Autodesk Inventor part; units mm, degrees
ref_plane "YZ Plane" through (0, 0, 0) normal (1, 0, 0) x (0, 1, 0)
ref_plane "XZ Plane" through (0, 0, 0) normal (0, 1, 0) x (-1, 0, 0)
ref_plane "XY Plane" through (0, 0, 0) normal (0, 0, 1) x (1, 0, 0)
sketch "Sketch1" plane through (0, 0, 0) normal (0, 1, 0) x (-1, 0, 0)
  circle A0 centre (0, 0) radius 41.5
  circle A1 centre (0, 0) radius 36.5
  dimension "d0" = 83
  dimension "d1" = 73
extrude "Extrusion1" add sketch "Sketch1" along normal blind 2
sketch "Sketch4" plane through (0, 0, 0) normal (0, -1, 0) x (1, 0, 0)
  line L0 (-2.5, -20) -> (-2.5, -41.5)
  line L1 (-2.5, -41.5) -> (2.5, -41.5)
  line L2 (2.5, -41.5) -> (2.5, -20)
  line L3 (3.2204, 53.4593) -> (-2.5, -41.5) construction
  line L4 (-3.2204, 53.4593) -> (2.5, -41.5) construction
  line L5 (2.5, -20) -> (-2.5, -20)
  line L6 (41.5, 2.5) -> (20, 2.5)
  line L7 (20, -2.5) -> (41.5, -2.5)
  line L8 (20, 2.5) -> (20, -2.5)
  line L9 (41.5, -2.5) -> (41.5, 2.5)
  line L10 (-2.5, 41.5) -> (-2.5, 20)
  line L11 (2.5, 20) -> (2.5, 41.5)
  line L12 (-2.5, 20) -> (2.5, 20)
  line L13 (2.5, 41.5) -> (-2.5, 41.5)
  line L14 (-41.5, -2.5) -> (-20, -2.5)
  line L15 (-20, 2.5) -> (-41.5, 2.5)
  line L16 (-20, -2.5) -> (-20, 2.5)
  line L17 (-41.5, 2.5) -> (-41.5, -2.5)
  point P0 (0, 0)
  dimension "d21" = 5
  dimension "d26" = 360
  dimension "d51" = 20
  dimension "d52" = 41.5
extrude "Extrusion3" add sketch "Sketch4" along normal blind 3
sketch "Sketch5" plane through (0, -3, 0) normal (0, -1, 0) x (1, 0, 0)
  arc A0 (-41.4246, 2.5) -> (2.5, -41.4246) centre (0, 0) ccw
  line L0 (2.5, -41.4246) -> (-2.5, -41.4246)
  line L1 (-2.5, -41.4246) -> (-2.5, -36.9246)
  line L2 (-2.5, -36.9246) -> (2.5, -36.9246)
  line L3 (2.5, -36.9246) -> (2.5, -41.4246)
  line L4 (41.4246, 2.5) -> (41.4246, -2.5)
  line L5 (41.4246, -2.5) -> (36.9246, -2.5)
  line L6 (36.9246, -2.5) -> (36.9246, 2.5)
  line L7 (36.9246, 2.5) -> (41.4246, 2.5)
  line L8 (-2.5, 41.4246) -> (2.5, 41.4246)
  line L9 (2.5, 41.4246) -> (2.5, 36.9246)
  line L10 (2.5, 36.9246) -> (-2.5, 36.9246)
  line L11 (-2.5, 36.9246) -> (-2.5, 41.4246)
  line L12 (-41.4246, -2.5) -> (-41.4246, 2.5)
  line L13 (-41.4246, 2.5) -> (-36.9246, 2.5)
  line L14 (-36.9246, 2.5) -> (-36.9246, -2.5)
  line L15 (-36.9246, -2.5) -> (-41.4246, -2.5)
  point P0 (0, -41.5)
  dimension "d30" = 5
  dimension "d31" = 4.5
  dimension "d34" = 360
extrude "Extrusion4" add sketch "Sketch5" along normal blind 40 contours L13 L14 L15 L12 | L1 L2 L3 L0 | L4 L5 L6 L7 | L8 L9 L10 L11
sketch "Sketch7" plane through (0, 2, 0) normal (0, 1, 0) x (1, 0, 0)
  circle A0 centre (0, -39) radius 1.5
  circle A1 centre (0, -44.5) radius 1.5
  circle A2 centre (38.5381, -22.25) radius 1.5
  circle A3 centre (33.775, -19.5) radius 1.5
  circle A4 centre (38.5381, 22.25) radius 1.5
  circle A5 centre (33.775, 19.5) radius 1.5
  circle A6 centre (0, 44.5) radius 1.5
  circle A7 centre (0, 39) radius 1.5
  circle A8 centre (-38.5381, 22.25) radius 1.5
  circle A9 centre (-33.775, 19.5) radius 1.5
  circle A10 centre (-38.5381, -22.25) radius 1.5
  circle A11 centre (-33.775, -19.5) radius 1.5
  point P0 (0, 0)
  dimension "d41" = 3
  dimension "d42" = 39
  dimension "d43" = 3
  dimension "d44" = 44.5
  dimension "d47" = 360
extrude "Extrusion6" cut sketch "Sketch7" against normal blind 10 contours A2 | A3 | A4 | A5 | A8 | A9 | A10 | A11
sketch "Sketch8" plane through (0, -43, 0) normal (0, -1, 0) x (1, 0, 0)
  line L0 (-2.5, 36.4143) -> (-2.5, 41.4246)
  arc A0 (0, -41.5) -> (2.5, -41.4246) centre (0, 0) ccw
  line L1 (-2.5, 41.4246) -> (2.5, 41.4246)
  line L2 (2.5, 41.4246) -> (2.5, -41.4246)
  line L3 (2.5, -41.4246) -> (-2.5, -41.4246)
  line L4 (-2.5, -41.4246) -> (-2.5, 41.4246)
  line L5 (-36.4143, -2.5) -> (-41.4246, -2.5)
  line L6 (36.4143, 2.5) -> (41.4246, 2.5)
  line L7 (-41.4246, -2.5) -> (41.4246, -2.5)
  line L8 (41.4246, -2.5) -> (41.4246, 2.5)
  line L9 (41.4246, 2.5) -> (-41.4246, 2.5)
  line L10 (-41.4246, 2.5) -> (-41.4246, -2.5)
extrude "Extrusion7" add sketch "Sketch8" along normal blind 5
properties part number "Bottom- Control Surfaces"
Work out the finished part from the listing and answer in its coordinate system (mm). A direction names the side the tool comes from. Coordinates: 2 decimals unless noted, no trailing zeros. Loops run counter-clockwise (first coordinate to the right, second up) from the corner with the lowest first, then second, coordinate; pieces in that order, holes last. Notation, with made-up numbers: (82.25, -40) - (99.25, -40) arc R32 ccw to (99.25, -12) - close; hole circle Ø9 at (-12.75, 57.5). An arc over 180 degrees is marked (long way). Use a Markdown table: item, result.
Item 1: Consider probe 1 along Z at (x, y) = (0, 1); probe 2 along X at (y, z) = (1.35, -19.5) (1 decimal). Determine where each line is inside the solid, lowest interval first. Write a range as from..to.
Evaluation:
| item | result |
|---|---|
| probe 1 | z = -41.5..-36.5, 36.5..41.5 |
| probe 2 | x = -36.6..-35.3, -32.3..-30.9, 30.9..32.3, 35.3..36.6 |
Item 2: The mould has two halves that part along Z. Classify faces 1 (the cylindrical face through (-34.881, 1.014, -20.514)), 2 (the flat face through (41.425, -25, 0)), 3 (the flat face through (-38, -31, -2.5)): +Z half, -Z half, draft (parallel to the pull), parting line (faces both ways), or undercut.
Evaluation:
| item | result |
|---|---|
| face 1 | undercut |
| face 2 | draft |
| face 3 | -Z half |
Item 3: Given pin 1 Ø3 at (y, z) = (-4, -30) entering from -X; pin 2 Ø1.5 at (x, z) = (1, 26.5) entering from +Y; pin 3 Ø1 at (x, z) = (-30, -21) entering from -Y, each flat-ended and moving along its own axis, determine where each tip first touches the part or whether it passes through.
Evaluation:
| item | result |
|---|---|
| pin 1 | stops at x = -2.5 |
| pin 2 | stops at y = 0 |
| pin 3 | stops at y = 0 |
Item 4: Find section D-D, the plane z = 14.5. Determine the outline of the cut face in (x, y), and give its area (3 significant figures).
Evaluation:
| item | result |
|---|---|
| outline | (-38.88, 0) - (-33.5, 0) - (-33.5, 2) - (-38.88, 2) - close; (-2.5, -48) - (2.5, -48) - (2.5, -43) - (-2.5, -43) - close; (33.5, 0) - (38.88, 0) - (38.88, 2) - (33.5, 2) - close |
| area | 46.6 mm2 |
Item 5: Find section C-C, the plane x = 10. Determine the outline of the cut face in (y, z).
Evaluation:
| item | result |
|---|---|
| outline | (-48, -2.5) - (-43, -2.5) - (-43, 2.5) - (-48, 2.5) - close; (0, -40.28) - (2, -40.28) - (2, -35.1) - (0, -35.1) - close; (0, 35.1) - (2, 35.1) - (2, 40.28) - (0, 40.28) - close |
Item 6: For faces 4 (the flat face through (-28, 0, 0)), 5 (the flat face through (38, -29, -2.5)), 6 (the flat face through (-29, -3, 0)), 7 (the flat face through (-38, -29, 2.5)), determine the directions among +Z, -Z, +X, -X, +Y, -Y from which every point of the face is accessible in a straight line to the end or side of a thin tool.
Evaluation:
| item | result |
|---|---|
| face 4 | +Y |
| face 5 | -Z, +X, -Y |
| face 6 | +Z, -Z |
| face 7 | +Z, -X, -Y |
Item 7: Find section B-B, the plane z = 24.5. Determine the outline of the cut face in (x, y), and give its area (3 significant figures).
Evaluation:
| item | result |
|---|---|
| outline | (-33.5, 0) - (-27.06, 0) - (-27.06, 2) - (-33.5, 2) - close; (-2.5, -48) - (2.5, -48) - (2.5, -43) - (-2.5, -43) - close; (-2.5, -3) - (2.5, -3) - (2.5, 0) - (-2.5, 0) - close; (27.06, 0) - (33.5, 0) - (33.5, 2) - (27.06, 2) - close |
| area | 65.8 mm2 |
Item 8: Find section A-A, the plane y = -22. Determine the outline of the cut face in (x, z), and give its area (3 significant figures).
Evaluation:
| item | result |
|---|---|
| outline | (-41.42, -2.5) - (-36.92, -2.5) - (-36.92, 2.5) - (-41.42, 2.5) - close; (-2.5, -41.42) - (2.5, -41.42) - (2.5, -36.92) - (-2.5, -36.92) - close; (-2.5, 36.92) - (2.5, 36.92) - (2.5, 41.42) - (-2.5, 41.42) - close; (36.92, -2.5) - (41.42, -2.5) - (41.42, 2.5) - (36.92, 2.5) - close |
| area | 90.0 mm2 |
